from build123d import *

# Parameters (mm, degrees)
SKETCH1_R           = 7.5
SKETCH1_R_2         = 5.125
BOSS_EXTRUDE1_DEPTH = 1
SKETCH2_R           = 6.5
SKETCH2_R_2         = 5.125
BOSS_EXTRUDE2_DEPTH = 3.5
CHAMFER1_SIZE       = 1


with BuildPart() as part:
    # Sketch1 → Boss-Extrude1 (new body)
    with BuildSketch(Plane.XY):
        Circle(SKETCH1_R)
        Circle(SKETCH1_R_2, mode=Mode.SUBTRACT)
    extrude(amount=BOSS_EXTRUDE1_DEPTH)

    # Sketch2 → Boss-Extrude2 (add)
    with BuildSketch(Plane.XY.offset(1)):
        Circle(SKETCH2_R)
        Circle(SKETCH2_R_2, mode=Mode.SUBTRACT)
    extrude(amount=BOSS_EXTRUDE2_DEPTH)

    # Chamfer1
    chamfer1_edges = [part.edges().sort_by_distance(p)[0] for p in [
        (-6.5, 0, 1),
    ]]
    chamfer(chamfer1_edges, length=CHAMFER1_SIZE - 0.0001)  # a hair under: the kernel refuses the full size

    # Mirror5: part across plane


with BuildPart() as part_1:
    add(part.part)
    add(part.part.mirror(Plane.XY.offset(4.5)))


solid = part_1.part
The model under review builds one solid part; all positions refer to its coordinate system, in mm. Give positions to 0.01 mm unless a question says otherwise; leave off trailing zeros. Order: outer loops, then holes, each group sorted by start corner. A loop starts at its lowest first (then second) coordinate and runs counter-clockwise, first axis right, second up. Notation, with made-up numbers: M 45.5,45.5 L 97.5,45.5 A14 cw 97.5,59.5 Z; hole C 31,-28 d7. An arc over 180 degrees is marked long. Answer in a Markdown table with one row per item. Add a question column.
1. For pin 1 Ø5 at (x, z) = (-2.5, 2.5) entering from +Y; pin 2 Ø2 at (x, z) = (5, 2) entering from +Y, all flat-tipped, find the tip position at first contact; note any pin that passes through.
2. Add section C-C on z = 6.75. State the section outline as (x, y) points (3 decimals).
3. To check wall thickness, follow line 1 along Y through (x, z) = (0, 6.75) (3 decimals); line 2 along Y through (x, z) = (-1, 1.5); line 3 along X through (y, z) = (-2.25, 4). State the ranges of each line that lie inside material, in increasing order.
The answers:
| question | item | result |
|---|---|---|
| 1 | pin 1 | y = 7.48 |
| 1 | pin 2 | y = 5.83 |
| 2 | outline | C 0,0 d13; hole C 0,0 d10.25 |
| 3 | line 1 | -6.5 to -5.125, 5.125 to 6.5 |
| 3 | line 2 | -6.93 to -5.03, 5.03 to 6.93 |
| 3 | line 3 | -6.1 to -4.6, 4.6 to 6.1 |
